Source: three-view drawing plus pictorial views. Frame: mm from the lowest corner of the part. A direction names the side the tool comes from. Coordinates: 2 decimals unless noted, no trailing zeros. Write each loop counter-clockwise with the first axis right and the second up, starting at its lowest first coordinate (ties: lowest second). Pieces come first, ordered by that corner, then holes. Notation, with made-up numbers: (-25, 2) -> (24, 2) arc R31 cw to (24, 30) -> close; hole circle Ø6 at (89, -21). An arc over 180 degrees is marked (long way). One line per item, written item: value.
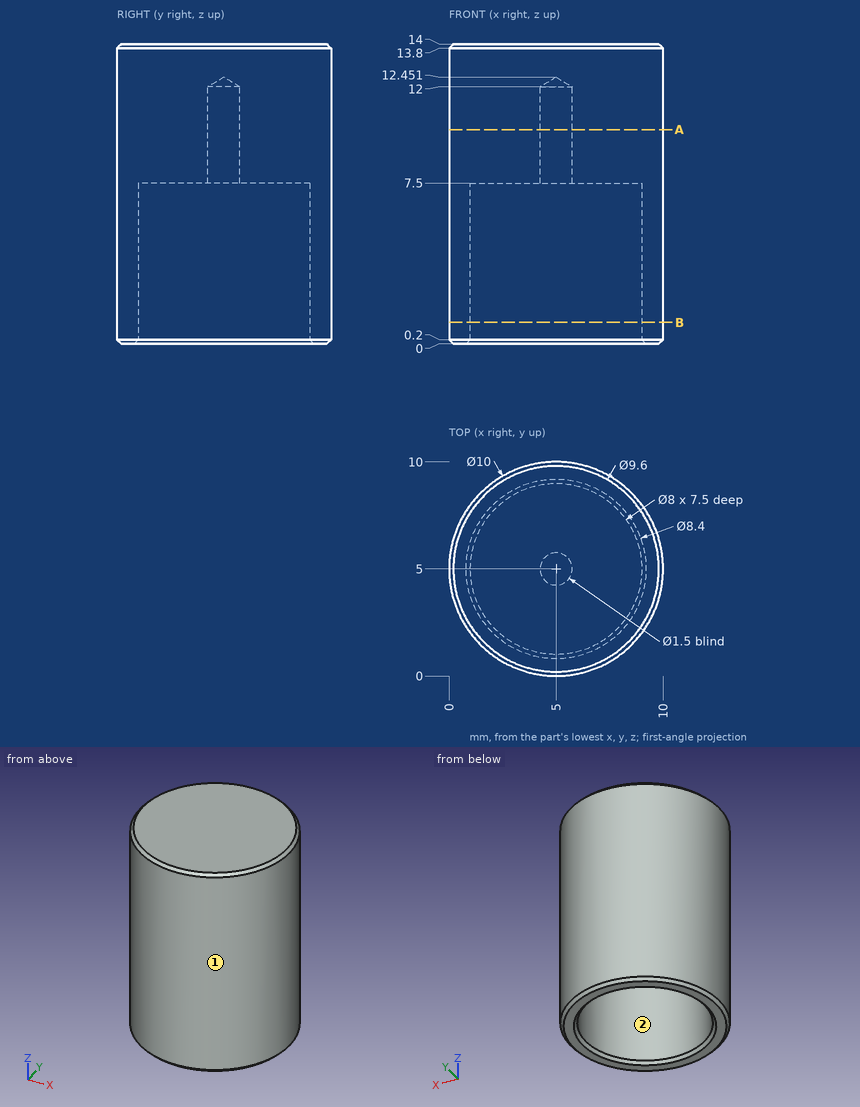
(1) Reachability of the marked faces 1 and 2 from +Z, -Z, +X, -X, +Y, -Y: full face, straight path, thin tool, end or side. Return the list, or none.
Responses:
face 1: +Z, -Z
face 2: -Z
(2) Section A-A (z = 10). Return the cut outline in (x, y).
Responses:
outline: circle Ø10 at (5, 5); hole circle Ø1.5 at (5, 5)
(3) Section B-B (z = 1). Return the cut outline in (x, y).
Responses:
outline: circle Ø10 at (5, 5); hole circle Ø8 at (5, 5)
(4) First-contact query: pin 1 (5 mm diameter, centred on x = 8, z = 2.5, fed in from -Y) (1 decimal); pin 2 (6 mm diameter, centred on y = 9, z = 4, fed in from -X). Flat tips, straight axial feed; report the tip coordinate or a pass-through.
Responses:
pin 1: stops at y = 0
pin 2: stops at x = 0.1
(5) Line query: line 1 (Y direction, x = 5, z = 8.85); line 2 (Y direction, x = 5, z = 6); line 3 (Z direction, x = 5.5, y = 6). Output: solid intervals per line, ascending. Write a range as [from, to].
Responses:
line 1: y = [0, 4.25], [5.75, 10]
line 2: y = [0, 1], [9, 10]
line 3: z = [7.5, 14]
